from build123d import *

# Parameters (mm, degrees)
SKETCH1_W           = 280.4
SKETCH1_H           = 12
BOSS_EXTRUDE1_DEPTH = 3
SKETCH3_R           = 1.5
CUT_EXTRUDE1_DEPTH  = 141.360393274
SKETCH6_W           = 140.2
SKETCH6_H           = 12
CUT_EXTRUDE2_DEPTH  = 141.360393274
SKETCH7_W           = 1.95
SKETCH7_H           = 1.95
BOSS_EXTRUDE2_DEPTH = 4
FILLET1_R           = 0.6


with BuildPart() as part:
    # Sketch1 → Boss-Extrude1 (new body)
    with BuildSketch(Plane(origin=(0, 0, 0), x_dir=(1, 0, 0), z_dir=(0, 1, 0))):
        Rectangle(SKETCH1_W, SKETCH1_H)
    extrude(amount=BOSS_EXTRUDE1_DEPTH)

    # Sketch3 → Cut-Extrude1 (cut, through all)
    with BuildSketch(Plane(origin=(0, 3, 0), x_dir=(1, 0, 0), z_dir=(0, 1, 0))):
        with Locations(Location((-136.25, 0, 0), (0, 0, 270))):
            Circle(SKETCH3_R)
        with Locations(Location((136.25, 0, 0), (0, 0, 270))):
            Circle(SKETCH3_R)
    extrude(amount=-CUT_EXTRUDE1_DEPTH, mode=Mode.SUBTRACT)

    # Sketch6 → Cut-Extrude2 (cut, through all)
    with BuildSketch(Plane(origin=(0, 3, 0), x_dir=(1, 0, 0), z_dir=(0, 1, 0))):
        with Locations((70.1, 0)):
            Rectangle(SKETCH6_W, SKETCH6_H)
    extrude(amount=-CUT_EXTRUDE2_DEPTH, mode=Mode.SUBTRACT)

    # Sketch7 → Boss-Extrude2 (add)
    with BuildSketch(Plane(origin=(0, 0, 0), x_dir=(0, 0, -1), z_dir=(1, 0, 0))):
        with Locations((0, 1.5)):
            Rectangle(SKETCH7_W, SKETCH7_H)
    extrude(amount=BOSS_EXTRUDE2_DEPTH)

    # Fillet1
    # the kernel refuses this fillet: 0.6 mm, written as the material it adds along each edge
    with BuildSketch(Plane(origin=(0, 0.525, -0.975), x_dir=(0, 0, -1), z_dir=(0, 1, 0)), Plane(origin=(0, 2.475, 0.975), x_dir=(0, 0, 1), z_dir=(0, -1, 0))) as fillet1_piece_1:
        with BuildLine():
            CenterArc((FILLET1_R, -FILLET1_R), FILLET1_R, 90, 90)
            Line((0, -FILLET1_R), (0, 0))
            Line((0, 0), (FILLET1_R, 0))
        make_face()
    fillet1_piece_1_solid = extrude(amount=1.95, mode=Mode.PRIVATE)
    with BuildSketch(Plane(origin=(0, 2.475, -0.975), x_dir=(0, 1, 0), z_dir=(0, 0, 1)), Plane(origin=(0, 0.525, 0.975), x_dir=(0, -1, 0), z_dir=(0, 0, -1))) as fillet1_piece_2:
        with BuildLine():
            CenterArc((0.6, -0.595294045), FILLET1_R, 97.180755781, 82.819244219)
            Line((0, -0.595294045), (0, 0))
            Line((0, 0), (0.525, 0))
        make_face()
    fillet1_piece_2_solid = extrude(amount=1.95, mode=Mode.PRIVATE)
    with BuildSketch(Plane(origin=(0, -0.975, -0.975), x_dir=(0, 0, -1), z_dir=(0, 1, 0))) as fillet1_piece_3a_section:
        with BuildLine():
            CenterArc((FILLET1_R, -FILLET1_R), FILLET1_R, 90, 90)
            Line((0, -FILLET1_R), (0, 0))
            Line((0, 0), (FILLET1_R, 0))
        make_face()
    fillet1_piece_3a = extrude(amount=3.45, mode=Mode.PRIVATE)
    fillet1_piece_3a = split(fillet1_piece_3a, bisect_by=Plane(origin=(0, 0, -0.975), z_dir=(0, 1, 0)), keep=Keep.TOP, mode=Mode.PRIVATE)
    fillet1_piece_3a = split(fillet1_piece_3a, bisect_by=Plane(origin=(0, 0.525, -0.975), z_dir=(0, -1, 0)), keep=Keep.TOP, mode=Mode.PRIVATE)
    with BuildSketch(Plane(origin=(0, 0.525, 0.975), x_dir=(0, -1, 0), z_dir=(0, 0, -1))) as fillet1_piece_3b_section:
        with BuildLine():
            CenterArc((0.6, -0.595294045), FILLET1_R, 97.180755781, 82.819244219)
            Line((0, -0.595294045), (0, 0))
            Line((0, 0), (0.525, 0))
        make_face()
    fillet1_piece_3b = extrude(amount=3.438235112, mode=Mode.PRIVATE)
    fillet1_piece_3b = split(fillet1_piece_3b, bisect_by=Plane(origin=(0, 0.525, -0.975), z_dir=(0, 0, -1)), keep=Keep.TOP, mode=Mode.PRIVATE)
    fillet1_piece_3 = fillet1_piece_3a & fillet1_piece_3b
    with BuildSketch(Plane(origin=(0, 2.475, -2.463235112), x_dir=(0, 1, 0), z_dir=(0, 0, 1))) as fillet1_piece_4a_section:
        with BuildLine():
            CenterArc((0.6, -0.595294045), FILLET1_R, 97.180755781, 82.819244219)
            Line((0, -0.595294045), (0, 0))
            Line((0, 0), (0.525, 0))
        make_face()
    fillet1_piece_4a = extrude(amount=3.438235112, mode=Mode.PRIVATE)
    fillet1_piece_4a = split(fillet1_piece_4a, bisect_by=Plane(origin=(0, 2.475, -0.975), z_dir=(0, 0, -1)), keep=Keep.TOP, mode=Mode.PRIVATE)
    with BuildSketch(Plane(origin=(0, 0.525, -0.975), x_dir=(0, 0, -1), z_dir=(0, 1, 0))) as fillet1_piece_4b_section:
        with BuildLine():
            CenterArc((FILLET1_R, -FILLET1_R), FILLET1_R, 90, 90)
            Line((0, -FILLET1_R), (0, 0))
            Line((0, 0), (FILLET1_R, 0))
        make_face()
    fillet1_piece_4b = extrude(amount=3.45, mode=Mode.PRIVATE)
    fillet1_piece_4b = split(fillet1_piece_4b, bisect_by=Plane(origin=(0, 3, -0.975), z_dir=(0, -1, 0)), keep=Keep.TOP, mode=Mode.PRIVATE)
    fillet1_piece_4b = split(fillet1_piece_4b, bisect_by=Plane(origin=(0, 2.475, -0.975), z_dir=(0, 1, 0)), keep=Keep.TOP, mode=Mode.PRIVATE)
    fillet1_piece_4 = fillet1_piece_4a & fillet1_piece_4b
    with BuildSketch(Plane(origin=(0, 3.975, 0.975), x_dir=(0, 0, 1), z_dir=(0, -1, 0))) as fillet1_piece_5a_section:
        with BuildLine():
            CenterArc((FILLET1_R, -FILLET1_R), FILLET1_R, 90, 90)
            Line((0, -FILLET1_R), (0, 0))
            Line((0, 0), (FILLET1_R, 0))
        make_face()
    fillet1_piece_5a = extrude(amount=3.45, mode=Mode.PRIVATE)
    fillet1_piece_5a = split(fillet1_piece_5a, bisect_by=Plane(origin=(0, 3, 0.975), z_dir=(0, -1, 0)), keep=Keep.TOP, mode=Mode.PRIVATE)
    fillet1_piece_5a = split(fillet1_piece_5a, bisect_by=Plane(origin=(0, 2.475, 0.975), z_dir=(0, 1, 0)), keep=Keep.TOP, mode=Mode.PRIVATE)
    with BuildSketch(Plane(origin=(0, 2.475, -0.975), x_dir=(0, 1, 0), z_dir=(0, 0, 1))) as fillet1_piece_5b_section:
        with BuildLine():
            CenterArc((0.6, -0.595294045), FILLET1_R, 97.180755781, 82.819244219)
            Line((0, -0.595294045), (0, 0))
            Line((0, 0), (0.525, 0))
        make_face()
    fillet1_piece_5b = extrude(amount=3.438235112, mode=Mode.PRIVATE)
    fillet1_piece_5b = split(fillet1_piece_5b, bisect_by=Plane(origin=(0, 2.475, 0.975), z_dir=(0, 0, 1)), keep=Keep.TOP, mode=Mode.PRIVATE)
    fillet1_piece_5 = fillet1_piece_5a & fillet1_piece_5b
    with BuildSketch(Plane(origin=(0, 2.475, 0.975), x_dir=(0, 0, 1), z_dir=(0, -1, 0))) as fillet1_piece_6a_section:
        with BuildLine():
            CenterArc((FILLET1_R, -FILLET1_R), FILLET1_R, 90, 90)
            Line((0, -FILLET1_R), (0, 0))
            Line((0, 0), (FILLET1_R, 0))
        make_face()
    fillet1_piece_6a = extrude(amount=3.45, mode=Mode.PRIVATE)
    fillet1_piece_6a = split(fillet1_piece_6a, bisect_by=Plane(origin=(0, 0, 0.975), z_dir=(0, 1, 0)), keep=Keep.TOP, mode=Mode.PRIVATE)
    fillet1_piece_6a = split(fillet1_piece_6a, bisect_by=Plane(origin=(0, 0.525, 0.975), z_dir=(0, -1, 0)), keep=Keep.TOP, mode=Mode.PRIVATE)
    with BuildSketch(Plane(origin=(0, 0.525, 2.463235112), x_dir=(0, -1, 0), z_dir=(0, 0, -1))) as fillet1_piece_6b_section:
        with BuildLine():
            CenterArc((0.6, -0.595294045), FILLET1_R, 97.180755781, 82.819244219)
            Line((0, -0.595294045), (0, 0))
            Line((0, 0), (0.525, 0))
        make_face()
    fillet1_piece_6b = extrude(amount=3.438235112, mode=Mode.PRIVATE)
    fillet1_piece_6b = split(fillet1_piece_6b, bisect_by=Plane(origin=(0, 0.525, 0.975), z_dir=(0, 0, 1)), keep=Keep.TOP, mode=Mode.PRIVATE)
    fillet1_piece_6 = fillet1_piece_6a & fillet1_piece_6b
    add([fillet1_piece_1_solid, fillet1_piece_2_solid, fillet1_piece_3, fillet1_piece_4, fillet1_piece_5, fillet1_piece_6])
    # the kernel refuses this fillet: 0.6 mm, written as the material it takes off along each edge
    with BuildSketch(Plane(origin=(4, -0.975, -0.975), x_dir=(0, 0, 1), z_dir=(0, 1, 0)), Plane(origin=(4, 2.475, -2.475), x_dir=(0, -1, 0), z_dir=(0, 0, 1)), Plane(origin=(4, 0.525, 2.475), x_dir=(0, 1, 0), z_dir=(0, 0, -1))) as fillet1_2_piece_1:
        with BuildLine():
            CenterArc((FILLET1_R, -FILLET1_R), FILLET1_R, 90, 90)
            Line((0, -FILLET1_R), (0, 0))
            Line((0, 0), (FILLET1_R, 0))
        make_face()
    fillet1_2_piece_1_solid = extrude(amount=4.95, mode=Mode.PRIVATE)
    with BuildSketch(Plane(origin=(4, 3.975, 0.975), x_dir=(-1, 0, 0), z_dir=(0, -1, 0))) as fillet1_2_piece_2:
        with BuildLine():
            CenterArc((FILLET1_R, FILLET1_R), FILLET1_R, 180, 90)
            Line((0, FILLET1_R), (0, 0))
            Line((0, 0), (FILLET1_R, 0))
        make_face()
    fillet1_2_piece_2_solid = extrude(amount=4.95, mode=Mode.PRIVATE)
    add([fillet1_2_piece_1_solid, fillet1_2_piece_2_solid], mode=Mode.SUBTRACT)


solid = part.part
Check sheet for the modelled part. Datum: model origin and axes. Units: mm. A direction names the side the tool comes from. Give positions to 0.01 mm unless a question says otherwise; leave off trailing zeros. Loops run counter-clockwise (first coordinate to the right, second up) from the corner with the lowest first, then second, coordinate; pieces in that order, holes last. Notation, with made-up numbers: M 9,58.25 L 63,58.25 A33 ccw 63,94.25 Z; hole C 67,24.25 d9. An arc over 180 degrees is marked long. Return JSON: item names as keys, results as strings. Group by question number.
1. Go/stop test with flat-tipped pins: pin 1 (1.5 mm diameter, centred on y = 1, z = 3, fed in from +X); pin 2 (1.6 mm diameter, centred on x = 2.5, z = -0.5, fed in from -Y) (3 decimals); pin 3 (1 mm diameter, centred on x = 1.5, z = -0.5, fed in from +Y) (3 decimals). Record where each tip stops, or that it passes through.
2. Cross-section at A-A on x = -136.25. Record the boundary of the cut face in (y, z), plus the area to 3 significant figures.
3. Cross-section at B-B on z = 4.75. Record the boundary of the cut face in (x, y), plus the area to 3 significant figures.
4. Thickness scan on L1, parallel to X at y = 1.4, z = 0; L2, parallel to Z at x = -136.25, y = 0.9; L3, parallel to X at y = 2.65, z = -1.25. Record the ranges inside material, lowest first.
5. Mould release check, pull along Z, two halves, no side actions. Record for faces 1 (the flat face through (-71, 1, 6)), 2 (the cylindrical face through (-134.763, 1.521, -0.195)), 3 (the flat face through (-71, 0, 0)): released by +Z, released by -Z, zero draft, split by the parting line, or undercut.
6. Tool access check on faces 4 (the flat face through (0, 2, 4)), 5 (the flat face through (0, 2, -4)), 6 (the flat face through (-71, 1, -6)). Record the directions out of +Z, -Z, +X, -X, +Y, -Y that give a thin tool (end or side, any length) a straight path to the whole face; none if there is none.
Return value:
{
 "1": {"pin 1": "x = 0", "pin 2": "y = 0.525", "pin 3": "y = 2.475"},
 "2": {"outline": "M 0,-6 L 3,-6 L 3,-1.5 L 0,-1.5 Z; M 0,1.5 L 3,1.5 L 3,6 L 0,6 Z", "area": "27.0 mm^2"},
 "3": {"outline": "M -140.2,0 L 0,0 L 0,3 L -140.2,3 Z", "area": "421 mm^2"},
 "4": {"L1": "-140.2 to -137.75, -134.75 to 4", "L2": "-6 to -1.5, 1.5 to 6", "L3": "-140.2 to -137.08, -135.42 to 0.1"},
 "5": {"face 1": "released by +Z", "face 2": "undercut", "face 3": "zero draft"},
 "6": {"face 4": "+Z, +X, +Y, -Y", "face 5": "-Z, +X, +Y, -Y", "face 6": "-Z, +X, -X, +Y, -Y"}
}
